Read the model definition and answer for the solid it produces. Units are mm, in the model's axes. A direction names the side the tool comes from. Give positions to 0.01 mm unless a question says otherwise; leave off trailing zeros. Order: outer loops, then holes, each group sorted by start corner. A loop starts at its lowest first (then second) coordinate and runs counter-clockwise, first axis right, second up. Notation, with made-up numbers: (57, 3.25) -> (61, 3.25) arc R22 ccw to (61, 19.25) -> close; hole circle Ø11 at (-25.5, -26.75). An arc over 180 degrees is marked (long way). Answer as CSV lines item,"result". Start each with the question number.
1) Find section B-B (z = 20.5). Determine the outline of the cut face in (x, y).
2) For faces 5 (the face through (0, 1, -13)), 6 (the face through (25.1, 8.45, 9.21)), 7 (the face through (-12.488, 0.55, -0.49)), 8 (the face through (-10, -8, 35)), determine the directions among +Z, -Z, +X, -X, +Y, -Y from which every point of the face is accessible in a straight line to the end or side of a thin tool.
3) The mould has two halves that part along Z. Classify faces 1 (the face through (12.497, -0.275, -0.175)), 2 (the face through (0, 1, 13)), 3 (the face through (4.774, 0.275, 12.497)), 4 (the face through (21.144, 0.703, 15.985)): +Z half, -Z half, draft (parallel to the pull), parting line (faces both ways), or undercut.
4) Flat-ended cylindrical pins translate along their axes: pin 1 Ø4 at (x, y) = (4.5, 8) entering from -Z; pin 2 Ø12 at (y, z) = (-3, -5) entering from +X; pin 3 Ø3 at (x, y) = (5.5, -2.5) entering from -Z. Find the tip coordinate at first contact, or state that the pin passes through.
5) Find section D-D (y = -6). Determine the outline of the cut face in (x, z).
6) Straight lines are drawn through the part: L1, parallel to Z at x = 32.5, y = 0; L2, parallel to Y at x = 11, z = 3. For each, find the intervals that lie inside material, in ascending order. Write a range as from..to.
7) Find section A-A (y = 0). Determine the outline of the cut face in (x, z), and give its area (4 significant figures).
```python
from build123d import *

# Parameters (mm, degrees)
SKETCH_1_R      = 16
SKETCH_1_R_2    = 12.5
EXTRUDE_1_DEPTH = 35
SKETCH_2_R      = 16
SKETCH_2_R_2    = 12.5
EXTRUDE_2_DEPTH = 35


with BuildPart() as part:
    # 草图1 → 凸台-拉伸1 (new body, symmetric)
    with BuildSketch(Plane.XY):
        Circle(SKETCH_1_R)
        Circle(SKETCH_1_R_2, mode=Mode.SUBTRACT)
    extrude(amount=EXTRUDE_1_DEPTH, both=True)

    # 草图2 → 凸台-拉伸2 (add)
    with BuildSketch(Plane(origin=(0, 0, 0), x_dir=(0, 0, -1), z_dir=(1, 0, 0))):
        Circle(SKETCH_2_R)
        Circle(SKETCH_2_R_2, mode=Mode.SUBTRACT)
    extrude(amount=EXTRUDE_2_DEPTH)


solid = part.part
```
Findings below:
1,outline,"circle Ø32 at (0, 0); hole circle Ø25 at (0, 0)"
2,face 5,"+Z, -Z"
2,face 6,"+X"
2,face 7,"none"
2,face 8,"+Z, +X, -X, +Y, -Y"
3,face 1,"undercut"
3,face 2,"draft"
3,face 3,"undercut"
3,face 4,"parting line"
4,pin 1,"z = -14.83"
4,pin 2,"x = 16"
4,pin 3,"z = -15.97"
5,outline,"(-14.83, -35) -> (-10.97, -35) -> (-10.97, 35) -> (-14.83, 35) -> close; (0, -14.83) -> (10.97, -14.83) -> (10.97, -35) -> (14.83, -35) -> (14.83, -14.83) -> (35, -14.83) -> (35, -10.97) -> (14.83, -10.97) -> (14.83, 10.97) -> (35, 10.97) -> (35, 14.83) -> (14.83, 14.83) -> (14.83, 35) -> (10.97, 35) -> (10.97, 14.83) -> (0, 14.83) -> (0, 10.97) -> (10.97, 10.97) -> (10.97, -10.97) -> (0, -10.97) -> close"
6,L1,"-16..-12.5, 12.5..16"
6,L2,"-15.72..-12.13, -11.62..-5.94, 5.94..11.62, 12.13..15.72"
7,outline,"(-16, -35) -> (-12.5, -35) -> (-12.5, 35) -> (-16, 35) -> close; (0, -16) -> (12.5, -16) -> (12.5, -35) -> (16, -35) -> (16, -16) -> (35, -16) -> (35, -12.5) -> (16, -12.5) -> (16, 12.5) -> (35, 12.5) -> (35, 16) -> (16, 16) -> (16, 35) -> (12.5, 35) -> (12.5, 16) -> (0, 16) -> (0, 12.5) -> (12.5, 12.5) -> (12.5, -12.5) -> (0, -12.5) -> close"
7,area,"710.5 mm²"
